Can you work these out from the model? Positions are in its coordinate system, mm. A direction names the side the tool comes from. Give positions to 0.01 mm unless a question says otherwise; leave off trailing zeros. Order: outer loops, then holes, each group sorted by start corner. A loop starts at its lowest first (then second) coordinate and runs counter-clockwise, first axis right, second up. Notation, with made-up numbers: M -18.75,79.5 L -2.75,79.5 A27 cw -2.75,98.5 Z; hole C 81,46 d6. An arc over 180 degrees is marked long. Answer as a JSON object with one key per item and string values.
```python
from build123d import *

# Parameters (mm, degrees)
SKETCH1_W           = 24.384
SKETCH1_H           = 24.384
BOSS_EXTRUDE1_DEPTH = 2.54
SKETCH2_R           = 9.144
BOSS_EXTRUDE2_DEPTH = 1.27
SKETCH3_R           = 2
CUT_EXTRUDE1_DEPTH  = 35.694019831


with BuildPart() as part:
    # Sketch1 → Boss-Extrude1 (new body)
    with BuildSketch(Plane(origin=(0, 0, 0), x_dir=(1, 0, 0), z_dir=(0, 1, 0))):
        with Locations((12.192, -12.192)):
            Rectangle(SKETCH1_W, SKETCH1_H)
    extrude(amount=BOSS_EXTRUDE1_DEPTH)

    # Sketch2 → Boss-Extrude2 (add)
    with BuildSketch(Plane(origin=(0, 2.54, 0), x_dir=(1, 0, 0), z_dir=(0, 1, 0))):
        with Locations(Location((12.192, -12.192, 0), (0, 0, 270))):
            Circle(SKETCH2_R)
    extrude(amount=BOSS_EXTRUDE2_DEPTH)

    # Sketch3 → Cut-Extrude1 (cut, through all)
    with BuildSketch(Plane(origin=(0, 3.81, 0), x_dir=(1, 0, 0), z_dir=(0, 1, 0))):
        with Locations(Location((12.192, -12.192, 0), (0, 0, 270))):
            Circle(SKETCH3_R)
    extrude(amount=-CUT_EXTRUDE1_DEPTH, mode=Mode.SUBTRACT)


solid = part.part
```
1) Thinking about a two-plate mould opening in Z: for faces 3 (the face through (6.628, 3.166, 4.936)), 4 (the face through (12, 0, 15)), 5 (the face through (13.544, 1.932, 10.718)), which applies, pulls with the +Z half, pulls with the -Z half, needs draft (parallel to the pull), parting line crosses it, or undercut?
Results found:
{"face 3": "parting line crosses it", "face 4": "needs draft", "face 5": "undercut"}
2) I need wall thicknesses on L1, parallel to Y at x = 1.75, z = 14; L2, parallel to X at y = 3.35, z = 4; L3, parallel to X at y = 3.5, z = 12.5. Which ranges of each line are inside material? Lowest first, please.
Results found:
{"L1": "y = 0 to 2.54", "L2": "x = 8.13 to 16.25", "L3": "x = 3.05 to 10.22, 14.17 to 21.33"}
3) I want a section at C-C on y = 0.6. Write out the boundary of the cut face in (x, z).
Results found:
{"outline": "M 0,0 L 24.38,0 L 24.38,24.38 L 0,24.38 Z; hole C 12.19,12.19 d4"}
4) I want a section at B-B on z = 12.75. Write out the boundary of the cut face in (x, y).
Results found:
{"outline": "M 0,0 L 10.27,0 L 10.27,3.81 L 3.07,3.81 L 3.07,2.54 L 0,2.54 Z; M 14.11,0 L 24.38,0 L 24.38,2.54 L 21.32,2.54 L 21.32,3.81 L 14.11,3.81 Z"}
5) For faces 1 (the face through (14.4, 3.81, 12.1)), 2 (the face through (17.4, 2.54, 20.1)), which set-ups out of +Z, -Z, +X, -X, +Y, -Y let a thin tool reach every point of the face, with its end or its side?
Results found:
{"face 1": "+Z, -Z, +X, -X, +Y", "face 2": "+Y"}
6) I want a section at D-D on z = 9. Write out the boundary of the cut face in (x, y).
Results found:
{"outline": "M 0,0 L 24.38,0 L 24.38,2.54 L 20.76,2.54 L 20.76,3.81 L 3.62,3.81 L 3.62,2.54 L 0,2.54 Z"}
7) I want a section at A-A on x = 12.75. Write out the boundary of the cut face in (y, z).
Results found:
{"outline": "M 0,0 L 2.54,0 L 2.54,3.07 L 3.81,3.07 L 3.81,10.27 L 0,10.27 Z; M 0,14.11 L 3.81,14.11 L 3.81,21.32 L 2.54,21.32 L 2.54,24.38 L 0,24.38 Z"}
